Source: CAD feature listing. Evaluate the final solid. Frame: model axes, mm. Coordinates: 2 decimals unless noted, no trailing zeros. Order: outer loops, then holes, each group sorted by start corner. A loop starts at its lowest first (then second) coordinate and runs counter-clockwise, first axis right, second up.
```python
from build123d import *

# Parameters (mm, degrees)
F1_DEPTH = 19.05
F3_DEPTH = 12.7
F4_SIZE  = 6.35


with BuildPart() as f1:
    # F0 (on Front) → F1 (new body)
    with BuildSketch(Plane.XZ):
        with BuildLine():
            Line((38.1, -12.7), (38.1, 12.7))
            Line((38.1, 12.7), (-38.1, 12.7))
            Line((-38.1, 12.7), (-38.1, 5.715))
            ThreePointArc((-38.1, 5.715), (-34.0588847455, 4.0411152545), (-32.385, 0))
            ThreePointArc((-32.385, 0), (-34.0588847455, -4.0411152545), (-38.1, -5.715))
            Line((-38.1, -5.715), (-38.1, -12.7))
            Line((-38.1, -12.7), (38.1, -12.7))
        make_face()
    extrude(amount=F1_DEPTH)

    # F2 (on face) → F3 (join)
    with BuildSketch(Plane(origin=(0, 0, 0), x_dir=(-1, 0, 0), z_dir=(0, 1, 0))):
        with BuildLine():
            add(Edge.make_bspline(
                [(-38.1, 12.7), (-19.05, 8.4666666667), (15.2730799035, 0.839315577), (-12.2449852881, -6.7880355127), (-26.9177044879, -10.182053269)],
                knots=[0, 0, 0, 0, 0.5, 0.9008682389, 0.9008682389, 0.9008682389, 0.9008682389], degree=3))
            Line((-38.1, 12.7), (-38.1, -12.7))
            add(Edge.make_bspline(
                [(-26.9177044879, -10.182053269), (-30.546159807, -11.021368846), (-34.3230799035, -11.860684423), (-38.1, -12.7)],
                knots=[0.9008682389, 0.9008682389, 0.9008682389, 0.9008682389, 1, 1, 1, 1], degree=3))
        make_face()
    extrude(amount=F3_DEPTH)

    # F4
    f4_edges = [f1.edges().sort_by_distance(p)[0] for p in [
        (38.1, 12.7, 0),
    ]]
    chamfer(f4_edges, length=F4_SIZE)


solid = f1.part
```
Q1. Section query A-A on y = -7. Output: boundary loops of the cut face in (x, z) (3 decimals), plus the area to 3 significant figures.
Solutions:
outline: (-38.1, -12.7) - (38.1, -12.7) - (38.1, 12.7) - (-38.1, 12.7) - (-38.1, 5.715) arc R5.715 cw to (-38.1, -5.715) - close
area: 1,880 mm2
Q2. Material intervals for line 1 along Y through (x, z) = (-3.5, -0.5); line 2 along X through (y, z) = (2.5, 2.25); line 3 along X through (y, z) = (-12.5, 1), sorted ascending.
Solutions:
line 1: y = -19.05 to 0
line 2: x = 1.69 to 38.1
line 3: x = -32.47 to 38.1
Q3. Section query B-B on x = -19.5. Output: boundary loops of the cut face in (y, z).
Solutions:
outline: (-19.05, -12.7) - (0, -12.7) - (0, 12.7) - (-19.05, 12.7) - close
Q4. Pull-direction query (Y, two-part tool) for faces 1 (the flat face through (38.1, -7, 0)), 2 (the flat face through (-1, -19.05, 0)), 3 (the flat face through (34.88, 9.57, 0.18)); classes: pulls with the +Y half, pulls with the -Y half, needs draft (parallel to the pull), parting line crosses it, or undercut.
Solutions:
face 1: needs draft
face 2: pulls with the -Y half
face 3: pulls with the +Y half
Q5. Pin query (flat end, axial travel): P1, Ø5, axis at y = -2, z = 1.5, coming from the -X side; P2, Ø12.5, axis at x = -16, z = 0, coming from the +Y side; P3, Ø5, axis at x = 21, y = 3, coming from the -Z side. Return the tip coordinate at first contact, or that it passes through.
Solutions:
P1: stops at x = -34.02
P2: stops at y = 0
P3: stops at z = -9.38
